Autodesk Inventor part; units mm, degrees
ref_plane "YZ Plane" through (0, 0, 0) normal (1, 0, 0) x (0, 1, 0)
ref_plane "XZ Plane" through (0, 0, 0) normal (0, 1, 0) x (-1, 0, 0)
ref_plane "XY Plane" through (0, 0, 0) normal (0, 0, 1) x (1, 0, 0)
sketch "Sketch1" plane through (0, 0, 0) normal (0, 1, 0) x (-1, 0, 0)
  line L0 (8, 0) -> (-48, 0)
  line L1 (0, -70) -> (0, 70)
  line L2 (-40, 50) -> (0, 50)
  line L3 (0, 50) -> (0, -50)
  line L4 (0, -50) -> (-40, -50)
  line L5 (-40, -50) -> (-40, 50)
  point P0 (0, 0)
  point P1 (0, 50)
  dimension "d0" = 40
  dimension "d1" = 100
extrude "Extrusion1" add sketch "Sketch1" against normal blind 3
sketch "Sketch2" plane through (0, -3, 0) normal (0, -1, 0) x (1, 0, 0)
  line L0 (0, -50) -> (40, -50)
  line L1 (40, -50) -> (40, 50)
  line L2 (40, 50) -> (0, 50)
  line L3 (0, 50) -> (0, -50)
  line L4 (40, 35) -> (0, 35)
  line L5 (40, -50) -> (40, 50)
  line L6 (40, -35) -> (0, -35)
  line L7 (40, 30) -> (0, 30)
  line L8 (40, -30) -> (0, -30)
  point P0 (0, 0)
  dimension "d4" = 15
  dimension "d5" = 15
  dimension "d6" = 5
  dimension "d7" = 5
extrude "Extrusion2" add sketch "Sketch2" along normal blind 21 contours L3 L8 L1 L6 | L3 L4 L1 L7
sketch "Sketch3" plane through (0, 0, 0) normal (0, 1, 0) x (1, 0, 0)
  line L0 (40, 50) -> (0, 50)
  line L1 (0, 50) -> (0, -50)
  line L2 (0, -50) -> (40, -50)
  line L3 (40, -50) -> (40, 50)
  line L4 (0, -44) -> (40, -44) construction
  arc A0 (12.5, -41.8) -> (12.5, -46.2) centre (12.5, -44) ccw
  arc A1 (27.5, -46.2) -> (27.5, -41.8) centre (27.5, -44) ccw
  line L5 (12.5, -41.8) -> (27.5, -41.8)
  line L6 (12.5, -46.2) -> (27.5, -46.2)
  line L7 (-8, 0) -> (48, 0)
  arc A2 (12.5, 46.2) -> (12.5, 41.8) centre (12.5, 44) ccw
  arc A3 (27.5, 41.8) -> (27.5, 46.2) centre (27.5, 44) ccw
  line L8 (12.5, 41.8) -> (27.5, 41.8)
  line L9 (12.5, 46.2) -> (27.5, 46.2)
  point P0 (0, 0)
  dimension "d10" = 6
  dimension "d11" = 4.4
  dimension "d12" = 4.4
  dimension "d13" = 15
  dimension "d14" = 12.5
extrude "Extrusion3" cut sketch "Sketch3" against normal blind 18 contours L5 A1 L6 A0 | L9 A3 L8 A2
sketch "Sketch4" plane through (0, -24, 0) normal (0, -1, 0) x (1, 0, 0)
  line L0 (40, 35) -> (-20, 35)
  line L1 (-20, 35) -> (-20, -35)
  line L2 (-20, -35) -> (40, -35)
  line L3 (40, -35) -> (40, 35)
  line L4 (40, 30) -> (40, 35)
  line L5 (40, 35) -> (0, 35)
  line L6 (0, 35) -> (0, 30)
  line L7 (0, 30) -> (40, 30)
  line L8 (0, -30) -> (0, -35)
  line L9 (0, -35) -> (40, -35)
  line L10 (40, -35) -> (40, -30)
  line L11 (40, -30) -> (0, -30)
  line L12 (40, 35) -> (0, 35)
  line L13 (0, -35) -> (40, -35)
  line L14 (40, -30) -> (40, 30)
  line L15 (40, -35) -> (40, -30)
  point P0 (0, 0)
  dimension "d18" = 20
extrude "Extrusion4" add sketch "Sketch4" against normal blind 3
sketch "Sketch5" plane through (0, 0, 0) normal (0, 1, 0) x (1, 0, 0)
  arc A0 (27.5, 41.8) -> (27.5, 46.2) centre (27.5, 44) ccw
  line L0 (27.5, 41.8) -> (12.5, 41.8)
  arc A1 (12.5, 46.2) -> (12.5, 41.8) centre (12.5, 44) ccw
  line L1 (12.5, 46.2) -> (27.5, 46.2)
  arc A2 (27.5, -46.2) -> (27.5, -41.8) centre (27.5, -44) ccw
  line L2 (27.5, -46.2) -> (12.5, -46.2)
  arc A3 (12.5, -41.8) -> (12.5, -46.2) centre (12.5, -44) ccw
  line L3 (12.5, -41.8) -> (27.5, -41.8)
  line L4 (40, 50) -> (0, 50)
  line L5 (0, 50) -> (0, -50)
  line L6 (0, -50) -> (40, -50)
  line L7 (40, -50) -> (40, 50)
  line L8 (-9.315, 0) -> (55.8902, 0)
  line L9 (40, -30) -> (0, -30)
  line L10 (0, 30) -> (40, 30)
  line L11 (40, -30) -> (40, 0) construction
  line L12 (40, 30) -> (40, 0) construction
  line L13 (0, -22) -> (30, -22)
  line L14 (30, -22) -> (30, 22)
  line L15 (30, 22) -> (0, 22)
  line L16 (0, 22) -> (0, -22)
  point P0 (0, 0)
  point P1 (0, 22)
  dimension "d30" = 44
  dimension "d31" = 10
extrude "Extrusion5" cut sketch "Sketch5" against normal up to surface (21 mm away) contours L15 L14 L8 L5 | L14 L13 L5 L8
sketch "Sketch6" plane through (40, -3, 50) normal (1, 0, 0) x (0, 0, -1)
  line L0 (0, 3) -> (100, 3)
  line L1 (0, 3) -> (0, 0)
  line L2 (15, 0) -> (0, 0)
  line L3 (15, 0) -> (15, -21)
  line L4 (85, -21) -> (15, -21)
  line L5 (85, 0) -> (85, -21)
  line L6 (100, 0) -> (85, 0)
  line L7 (100, 3) -> (100, 0)
  line L8 (80, 0) -> (20, 0)
  line L9 (80, 0) -> (80, -18)
  line L10 (20, -18) -> (80, -18)
  line L11 (20, 0) -> (20, -18)
  line L12 (85, 0) -> (85, -21)
  line L13 (100, 0) -> (85, 0)
  line L14 (0, 0) -> (15, 0)
  line L15 (3.8, 3) -> (3.8, 0)
  line L16 (15, -21) -> (15, 0)
  line L17 (0, 0) -> (15, -9)
  line L18 (15, 0) -> (15, -21)
  line L19 (100, 0) -> (85, -9)
  line L20 (85, 0) -> (85, -21)
  point P0 (50, 3)
  dimension "d53" = 12
  dimension "d54" = 12
extrude "Extrusion6" add sketch "Sketch6" against normal blind 3 contours L2 L3 L17 | L19 L5 L6
fillet "Fillet1" radius 8 4 edges at (30, -1.5, 22) (30, -1.5, -22) (0, -1.5, -22) (0, -1.5, 22)
chamfer "Chamfer1" distance 20 angle 45 2 edges at (-20, -22.5, -35) (-20, -22.5, 35)
sketch "Sketch9" plane through (0, -21, 0) normal (0, 1, 0) x (1, 0, 0)
  line L0 (-32, 0) -> (52, 0)
  line L1 (0, 70) -> (0, -70)
  line L2 (-20, 15) -> (-20, -15)
  arc A0 (-15, -7.5) -> (-11, -7.5) centre (-13, -7.5) ccw
  arc A1 (-11, 7.5) -> (-15, 7.5) centre (-13, 7.5) ccw
  line L3 (-13, -15) -> (-13, 15) construction
  line L4 (-15, -7.5) -> (-15, 7.5)
  line L5 (-11, -7.5) -> (-11, 7.5)
  arc A2 (25, -7.5) -> (29, -7.5) centre (27, -7.5) ccw
  arc A3 (29, 7.5) -> (25, 7.5) centre (27, 7.5) ccw
  line L6 (25, -7.5) -> (25, 7.5)
  line L7 (29, -7.5) -> (29, 7.5)
  point P0 (0, 0)
  dimension "d36" = 4
  dimension "d37" = 4
  dimension "d38" = 15
  dimension "d40" = 7
  dimension "d41" = 7.5
  dimension "d42" = 4
  dimension "d43" = 4
  dimension "d44" = 15
  dimension "d45" = 40
  dimension "d46" = 7.5
extrude "Extrusion9" cut sketch "Sketch9" against normal blind 10
fillet "Fillet2" radius 8 1 edges at (0, -1.5, -50)
fillet "Fillet3" radius 8 1 edges at (0, -1.5, 50)
fillet "Fillet4" radius 3 8 edges at (20, -21, -30) (0, -21, -32.5) (20, -21, 30) (0, -21, 32.5) (18.5, -3, 35) (20, -3, 30) (18.5, -3, -35) (20, -3, -30)
properties part number "soporte infe"
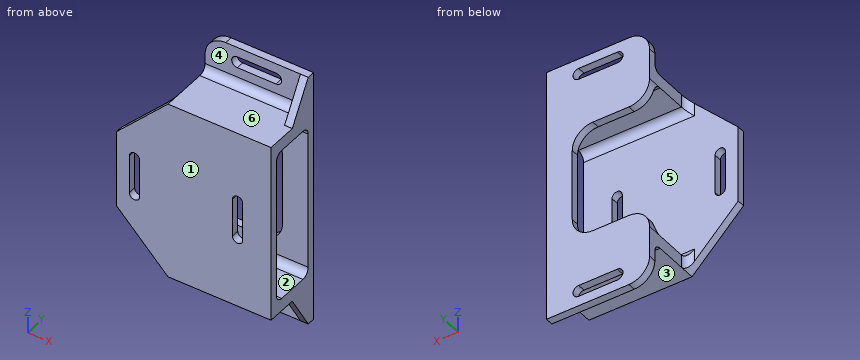
Read the model definition and answer for the solid it produces. Units are mm, in the model's axes. Face numbers are marked on the shaded views. A direction names the side the tool comes from. Round coordinates to 2 decimals unless told otherwise and drop trailing zeros. Order: outer loops, then holes, each group sorted by start corner. A loop starts at its lowest first (then second) coordinate and runs counter-clockwise, first axis right, second up.
1) The mould has two halves that part along Z. Classify the marked faces 4, 5 and 6: released by +Z, released by -Z, zero draft, split by the parting line, or undercut.
2) The part is cut by section D-D on y = -13. Write down the section's boundary in (x, z).
3) The part is cut by section B-B on x = 20.5. Give the number of separate pieces and of enclosed holes in the cut face, plus the area to 3 significant figures.
4) The part is cut by section A-A on y = -1.75. Write down the section's boundary in (x, z).
5) Flat-ended cylindrical pins translate along their axes: pin 1 (3.5 mm diameter, centred on x = 26.5, y = -14.5, fed in from +Z); pin 2 (2.5 mm diameter, centred on y = -9, z = 39, fed in from -X); pin 3 (6 mm diameter, centred on x = 17.5, y = -14, fed in from -Z). Find the tip coordinate at first contact, or state that the pin passes through.
6) The part is cut by section C-C on z = 16. Write down the section's boundary in (x, y), plus the area to 3 significant figures.
7) Straight lines are drawn through the part: L1, parallel to Z at x = 4, y = -16.75; L2, parallel to Y at x = 32, z = 10.5; L3, parallel to Z at x = 26, y = -5.25. For each, find the intervals that lie inside material, in ascending order.
8) For the marked faces 1, 2 and 3, determine the directions among +Z, -Z, +X, -X, +Y, -Y from which every point of the face is accessible in a straight line to the end or side of a thin tool.
Resolved:
1. face 4: zero draft
1. face 5: undercut
1. face 6: released by +Z
2. outline: (0, -35) - (40, -35) - (40, -30) - (0, -30) - close; (0, 30) - (40, 30) - (40, 35) - (0, 35) - close
3. separate pieces: 3
3. enclosed holes: 0
3. area: 543 mm2
4. outline: (0, -42) arc R8 ccw to (8, -50) - (40, -50) - (40, 50) - (8, 50) arc R8 ccw to (0, 42) - (0, 30) arc R8 ccw to (8, 22) - (22, 22) arc R8 cw to (30, 14) - (30, -14) arc R8 cw to (22, -22) - (8, -22) arc R8 ccw to (0, -30) - close; hole (12.5, -46.2) - (27.5, -46.2) arc R2.2 ccw to (27.5, -41.8) - (12.5, -41.8) arc R2.2 ccw to start; hole (12.5, 41.8) - (27.5, 41.8) arc R2.2 ccw to (27.5, 46.2) - (12.5, 46.2) arc R2.2 ccw to start
5. pin 1: stops at z = 35
5. pin 2: stops at x = 37
5. pin 3: stops at z = -35
6. outline: (-19, -24) - (40, -24) - (40, -21) - (-19, -21) - close; (29.75, -3) - (40, -3) - (40, 0) - (29.75, 0) - close
6. area: 208 mm2
7. L1: z = -35 to -30, 30 to 35
7. L2: y = -24 to -21, -3 to 0
7. L3: z = -35.1 to -29.9, 29.9 to 35.1
8. face 1: +Z, -Z, +X, -X, -Y
8. face 2: +X, -X
8. face 3: -Z, -X, -Y
